Answer from the drawing. Dimensions are ordinates in mm from the lowest x, y and z of the part. Round coordinates to 2 decimals unless told otherwise and drop trailing zeros. Order: outer loops, then holes, each group sorted by start corner. A loop starts at its lowest first (then second) coordinate and runs counter-clockwise, first axis right, second up.
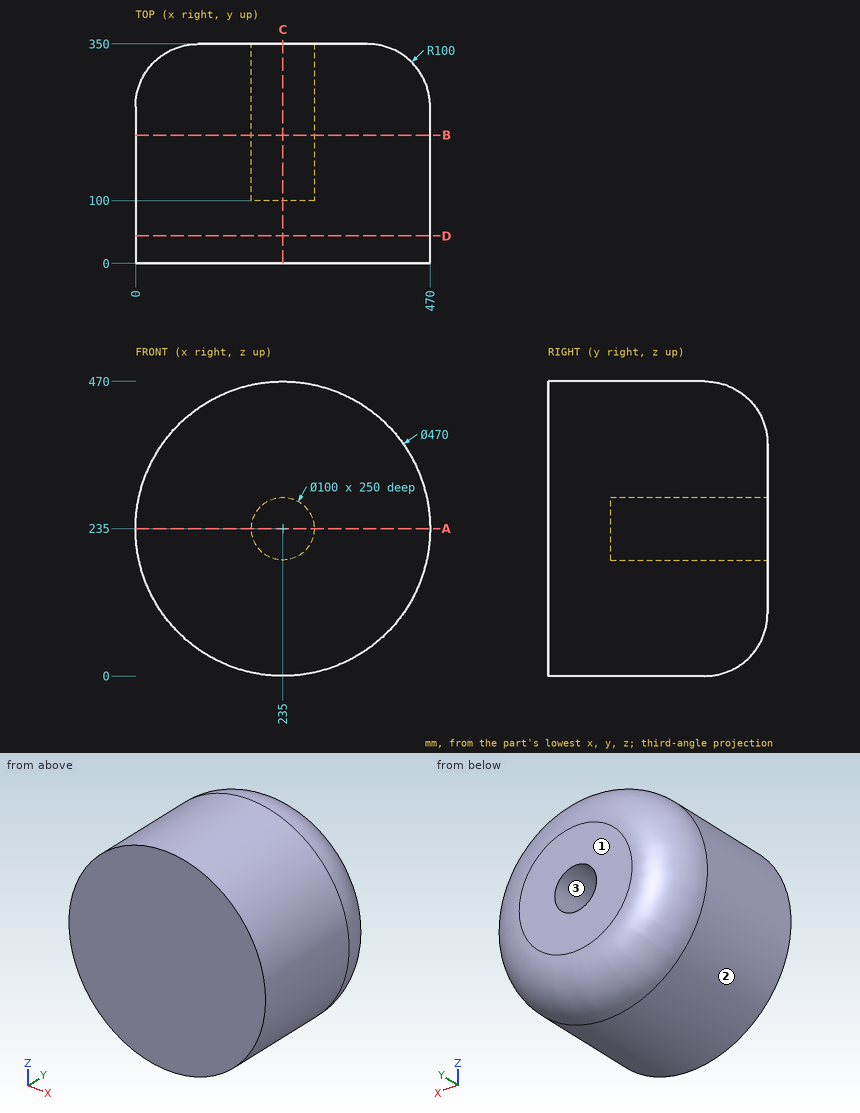
Q1. A cutting plane is placed at B-B, the plane y = 204.5. Give the vertices of the cut face in (x, z).
Outcome:
outline: circle Ø470 at (235, 235); hole circle Ø100 at (235, 235)
Q2. A cutting plane is placed at D-D, the plane y = 44. Give the vertices of the cut face in (x, z), plus the area to 3 significant figures.
Outcome:
outline: circle Ø470 at (235, 235)
area: 173,000 mm2
Q3. For a pull along Z with two mould halves and no side action, classify the marked faces 1, 2 and 3 as released by +Z, released by -Z, zero draft, split by the parting line, or undercut.
Outcome:
face 1: zero draft
face 2: split by the parting line
face 3: undercut
Q4. Straight lines are drawn through the part: probe 1 along X at (y, z) = (206, 235); probe 2 along X at (y, z) = (146, 246.5). For each, find the intervals that lie inside material, in ascending order.
Outcome:
probe 1: x = 0 to 185, 285 to 470
probe 2: x = 0.28 to 186.34, 283.66 to 469.72
Q5. A cutting plane is placed at C-C, the plane x = 235. Give the vertices of the cut face in (y, z), plus the area to 3 significant figures.
Outcome:
outline: (0, 0) - (250, 0) arc R100 ccw to (350, 100) - (350, 185) - (100, 185) - (100, 285) - (350, 285) - (350, 370) arc R100 ccw to (250, 470) - (0, 470) - close
area: 135,000 mm2
Q6. A cutting plane is placed at A-A, the plane z = 235. Give the vertices of the cut face in (x, y).
Outcome:
outline: (0, 0) - (470, 0) - (470, 250) arc R100 ccw to (370, 350) - (285, 350) - (285, 100) - (185, 100) - (185, 350) - (100, 350) arc R100 ccw to (0, 250) - close
Q7. Flat-ended cylindrical pins translate along their axes: pin 1 (4 mm diameter, centred on y = 198, z = 206.5, fed in from +X); pin 2 (6 mm diameter, centred on y = 61, z = 218, fed in from -X); pin 3 (5 mm diameter, centred on x = 413.5, y = 312.5, fed in from +Z). Find the tip coordinate at first contact, or state that the pin passes through.
Outcome:
pin 1: stops at x = 468.5
pin 2: stops at x = 0.42
pin 3: stops at z = 356.46
